Build history of the part. All positions in model axes, mm. A direction names the side the tool comes from. Round coordinates to 2 decimals unless told otherwise and drop trailing zeros. Loops run counter-clockwise (first coordinate to the right, second up) from the corner with the lowest first, then second, coordinate; pieces in that order, holes last. Notation, with made-up numbers: (58.5, 48) - (100.5, 48) arc R35 ccw to (100.5, 87) - close; hole circle Ø7 at (73.25, 27). An arc over 180 degrees is marked (long way). Put each result on its own line as item: value. Start each with the question number.
from build123d import *

# Parameters (mm, degrees)
ESQUISSE2_W             = 150
ESQUISSE2_H             = 55
BOSS_EXTRU_1_DEPTH      = 5
ESQUISSE3_W             = 150
ESQUISSE3_H             = 5
BOSS_EXTRU_2_DEPTH      = 30
BOSS_EXTRU_3_DEPTH      = 55
ENL_V_MAT_EXTRU_1_DEPTH = 164.554272338


with BuildPart() as part:
    # Esquisse2 → Boss.-Extru.1 (new body)
    with BuildSketch(Plane(origin=(0, 0, 0), x_dir=(1, 0, 0), z_dir=(0, 1, 0))):
        with Locations((75, 27.5)):
            Rectangle(ESQUISSE2_W, ESQUISSE2_H)
    extrude(amount=BOSS_EXTRU_1_DEPTH)

    # Esquisse3 → Boss.-Extru.2 (add)
    with BuildSketch(Plane(origin=(0, 5, 0), x_dir=(1, 0, 0), z_dir=(0, 1, 0))):
        with Locations((75, 2.5)):
            Rectangle(ESQUISSE3_W, ESQUISSE3_H)
        with Locations((75, 52.5)):
            Rectangle(ESQUISSE3_W, ESQUISSE3_H)
    extrude(amount=BOSS_EXTRU_2_DEPTH)

    # Esquisse4 → Boss.-Extru.3 (add)
    with BuildSketch(Plane.XY):
        Polygon((0, 0), (5.879626117, -12.608898898), (15.841573098, -11.73734147), (10.368360884, 0), align=None)
        Polygon((150, 0), (140.038053019, -0.871557427), (139.631639116, 0), align=None)
    extrude(amount=-BOSS_EXTRU_3_DEPTH)

    # Esquisse5 → Enlèv. mat.-Extru.1 (cut, through all)
    with BuildSketch(Plane.XY):
        Polygon((150, 0), (146.937896777, 35), (150, 35), align=None)
    extrude(amount=-ENL_V_MAT_EXTRU_1_DEPTH, mode=Mode.SUBTRACT)


solid = part.part
1) Which spindle directions (+Z, -Z, +X, -X, +Y, -Y) get a long thin tool onto all of the face, cutting with end or side? Do faces 4 (the face through (74, 20, -5)), 5 (the face through (74, 17, -55)). Say none if no direction does.
2) Slice it at B-B, the plane x = 98. Write the cut outline in (y, z), and give its area (3 significant figures).
3) Pull direction Y, two halves, no side cores. Call faces 1 (the face through (13.143, -5.951, -27.115)), 2 (the face through (145.09, -0.43, -27.12)), 3 (the face through (0, 4, -25)): pulls with the +Y half, pulls with the -Y half, needs draft (parallel to the pull), parting line crosses it, or undercut.
4) Drill centre lines: line 1 (Z direction, x = 31, y = 30); line 2 (Y direction, x = 135, z = -33.5); line 3 (Y direction, x = 134.5, z = -52). Where is each one in solid material? Low to high. Write a range as [from, to].
5) Slice it at A-A, the plane z = -2.5. Write the cut outline in (x, y).
6) Slice it at C-C, the plane y = 27. Write the cut outline in (x, z), and give its area (3 significant figures).
7) Drop flat-ended pins along their axis: pin 1 Ø8 at (x, z) = (97.5, -15) entering from +Y; pin 2 Ø3 at (x, z) = (124.5, -19) entering from -Y. Give the stop position or say it passes through.
8) Slice it at D-D, the plane y = 13. Write the cut outline in (x, z).
Taken from the geometry:
1. face 4: +X, -X, +Y
1. face 5: -Z, +X, -X, +Y, -Y
2. outline: (0, -55) - (35, -55) - (35, -50) - (5, -50) - (5, -5) - (35, -5) - (35, 0) - (0, 0) - close
2. area: 575 mm2
3. face 1: undercut
3. face 2: pulls with the -Y half
3. face 3: needs draft
4. line 1: z = [-55, -50], [-5, 0]
4. line 2: y = [0, 5]
4. line 3: y = [0, 35]
5. outline: (0, 0) - (5.88, -12.61) - (15.84, -11.74) - (10.37, 0) - (139.63, 0) - (140.04, -0.87) - (150, 0) - (146.94, 35) - (0, 35) - close
6. outline: (0, -55) - (147.64, -55) - (147.64, -50) - (0, -50) - close; (0, -5) - (147.64, -5) - (147.64, 0) - (0, 0) - close
6. area: 1,480 mm2
7. pin 1: stops at y = 5
7. pin 2: stops at y = 0
8. outline: (0, -55) - (148.86, -55) - (148.86, -50) - (0, -50) - close; (0, -5) - (148.86, -5) - (148.86, 0) - (0, 0) - close
